from build123d import *

# Parameters (mm, degrees)
F0_R     = 8
F1_DEPTH = 1
F2_R     = 5.75
F3_DEPTH = 1
F4_R     = 4.2
F5_DEPTH = 3
F6_R     = 0.75


with BuildPart() as f1:
    # F0 (on Top) → F1 (new body)
    with BuildSketch(Plane.XY):
        Circle(F0_R)
    extrude(amount=F1_DEPTH)

    # F2 (on face) → F3 (join)
    with BuildSketch(Plane.XY.offset(1)):
        Circle(F2_R)
    extrude(amount=F3_DEPTH)

    # F4 (on face) → F5 (join)
    with BuildSketch(Plane.XY.offset(2)):
        Circle(F4_R)
    extrude(amount=F5_DEPTH)

    # F6
    f6_edges = [f1.edges().sort_by_distance(p)[0] for p in [
        (-8, 0, 0),
    ]]
    fillet(f6_edges, radius=F6_R)


solid = f1.part
Could you check a few things on this model? Use its own coordinates, in mm. A direction names the side the tool comes from. Round coordinates to 2 decimals unless told otherwise and drop trailing zeros. Loops run counter-clockwise (first coordinate to the right, second up) from the corner with the lowest first, then second, coordinate; pieces in that order, holes last. Notation, with made-up numbers: (42, 31) - (68, 31) arc R25 ccw to (68, 50) - close; hole circle Ø5 at (88, 75.5). An arc over 180 degrees is marked (long way). Write item = value, one per line.
1) Imagine slicing it at A-A (y = 0). Please give me the cut outline in (x, z).
Computed:
outline = (-8, 0.75) arc R0.75 ccw to (-7.25, 0) - (7.25, 0) arc R0.75 ccw to (8, 0.75) - (8, 1) - (5.75, 1) - (5.75, 2) - (4.2, 2) - (4.2, 5) - (-4.2, 5) - (-4.2, 2) - (-5.75, 2) - (-5.75, 1) - (-8, 1) - close
2) I need wall thicknesses on line 1 along Z through (x, y) = (1, -4.25); line 2 along Z through (x, y) = (0, 6.5); line 3 along X through (y, z) = (2, 3.85). Which ranges of each line are inside material? Lowest first, please. Write a range as from..to.
Computed:
line_1 = 0..2
line_2 = 0..1
line_3 = -3.69..3.69
3) On a 3-axis mill with a long thin cutter (end or side, diameter ignored), from which of +Z, -Z, +X, -X, +Y, -Y can I reach the whole of each face in a straight line? I mean faces 1 (the cylindrical face through (4.006, 1.262, 3.479)), 2 (the flat face through (0, 0, 0)). Say none if no direction works.
Computed:
face_1 = +Z
face_2 = -Z, +X, -X, +Y, -Y
4) Imagine slicing it at C-C (z = 1.25). Please give me the cut outline in (x, y), and give its area (3 significant figures).
Computed:
outline = circle Ø11.5 at (0, 0)
area = 104 mm2
5) I'm going to push flat-ended pins straight in: P1, Ø1.5, axis at x = -5.5, z = 2, coming from the +Y side; P2, Ø1.5, axis at x = -1.5, z = 2, coming from the +Y side. Where does each tip first touch, or does it pass through?
Computed:
P1 = 3.24
P2 = 5.7
6) Imagine slicing it at D-D (z = 2.4). Please give me the cut outline in (x, y).
Computed:
outline = circle Ø8.4 at (0, 0)
